from build123d import *

# Parameters (mm, degrees)
SKETCH1_R           = 30
BOSS_EXTRUDE1_DEPTH = 427.485478
SKETCH2_R           = 25.004464226
CUT_EXTRUDE1_DEPTH  = 430.585653742


with BuildPart() as part:
    # Sketch1 → Boss-Extrude1 (new body)
    with BuildSketch(Plane(origin=(0, 0, 0), x_dir=(1, 0, 0), z_dir=(0, 1, 0))):
        with Locations(Location((0, 0, 0), (0, 0, 270))):
            Circle(SKETCH1_R)
    extrude(amount=BOSS_EXTRUDE1_DEPTH)

    # Sketch2 → Cut-Extrude1 (cut, through all)
    with BuildSketch(Plane(origin=(0, 0, 0), x_dir=(1, 0, 0), z_dir=(0, 1, 0))):
        with Locations(Location((0, 0, 0), (0, 0, 270))):
            Circle(SKETCH2_R)
    extrude(amount=CUT_EXTRUDE1_DEPTH, mode=Mode.SUBTRACT)

    # Chamfer1: read off the stored shape, not the designer's step
    # Chamfer1 outline → Chamfer1 (revolve, cut)
    with BuildSketch(Plane.XY):
        Polygon((30, 422.288826614), (30, 427.485477895), (25.004464226, 427.485477895), (25.004464226, 425.173000538), align=None)
        Polygon((30, 9.000864049), (25.004464226, 0.348342277), (25.004464226, 0), (30, 0), align=None)
    revolve(axis=Axis((0, 0, 0), (0, 1, 0)), mode=Mode.SUBTRACT)


solid = part.part
Read the model definition and answer for the solid it produces. Units are mm, in the model's axes. Coordinates: 2 decimals unless noted, no trailing zeros. Loops run counter-clockwise (first coordinate to the right, second up) from the corner with the lowest first, then second, coordinate; pieces in that order, holes last.
Q1. The part is cut by section B-B on z = 0. Write down the section's boundary in (x, y), and give its area (3 significant figures).
Q2. Each of these flat-tipped pins is pushed along its axis until it touches: pin 1 Ø6 at (x, y) = (-13, 180) entering from -Z; pin 2 Ø1.5 at (x, y) = (22, 57.5) entering from -Z; pin 3 Ø4 at (x, y) = (-5, 73) entering from -Z. Where does it stop, or does it pass through?
Q3. The part is cut by section A-A on x = 0. Write down the section's boundary in (y, z).
Q4. Consider probe 1 along X at (y, z) = (240, 0); probe 2 along X at (y, z) = (343, 14.5); probe 3 along Z at (x, y) = (8, 199). Determine where each line is inside the solid, lowest interval first.
Q5. The part is cut by section C-C on y = 56. Write down the section's boundary in (x, z), and give its area (3 significant figures).
Q6. The mould has two halves that part along Z. Classify faces 1 (the face through (7.51, 209.79, 23.85)), 2 (the face through (-5.5, 425, 24.7)): +Z half, -Z half, draft (parallel to the pull), parting line (faces both ways), or undercut.
Results below:
1. outline: (-30, 9) - (-25, 0.35) - (-25, 425.17) - (-30, 422.29) - close; (25, 0.35) - (30, 9) - (30, 422.29) - (25, 425.17) - close
1. area: 4,190 mm2
2. pin 1: stops at z = -28.28
2. pin 2: stops at z = -21.18
2. pin 3: stops at z = -29.85
3. outline: (0.35, -25) - (9, -30) - (422.29, -30) - (425.17, -25) - close; (0.35, 25) - (425.17, 25) - (422.29, 30) - (9, 30) - close
4. probe 1: x = -30 to -25, 25 to 30
4. probe 2: x = -26.26 to -20.37, 20.37 to 26.26
4. probe 3: z = -28.91 to -23.69, 23.69 to 28.91
5. outline: circle Ø60 at (0, 0); hole circle Ø50.01 at (0, 0)
5. area: 863 mm2
6. face 1: undercut
6. face 2: parting line
